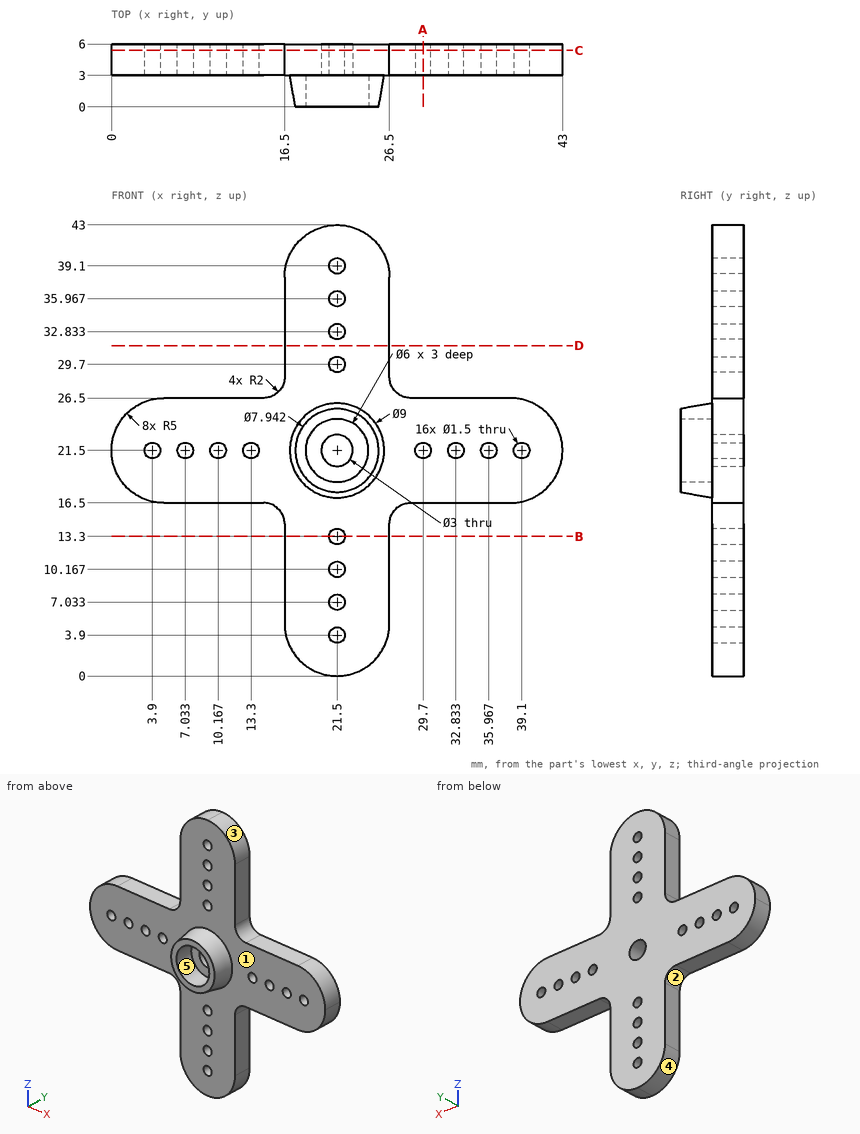
Verification items for this drawing (mm, ordinates from the low corner). A direction names the side the tool comes from. Round coordinates to 2 decimals unless told otherwise and drop trailing zeros. Write each loop counter-clockwise with the first axis right and the second up, starting at its lowest first coordinate (ties: lowest second). Pieces come first, ordered by that corner, then holes. Notation, with made-up numbers: M -8,0.5 L 29,0.5 A22 cw 29,31.5 Z; hole C 72.25,-11 d4. An arc over 180 degrees is marked long. Write item = value, one per line. Start each with the question number.
1. Gauge pin test, flat ends, axial feed: pin 1 (2 mm diameter, centred on y = 1.5, z = 35, fed in from -X); pin 2 (0.9 mm diameter, centred on y = 5, z = 10.5, fed in from +X); pin 3 (21.5 mm diameter, centred on x = 22, z = 18, fed in from -Y); pin 4 (5 mm diameter, centred on x = 21.5, z = 21.5, fed in from -Y). Record the tip position at first contact, or that the pin passes through.
2. Section check C-C, the plane y = 5.4. State how many separate pieces and enclosed holes the cut face has, then the cut area to 3 significant figures.
3. Section check A-A, the plane x = 29.7. Record the cut outline in (y, z), then the cut area to 3 significant figures.
4. Tool access check on the marked faces 1 and 2. Record the directions out of +Z, -Z, +X, -X, +Y, -Y that give a thin tool (end or side, any length) a straight path to the whole face; none if there is none.
5. Release check for a two-part mould opening along X. For the marked faces 3, 4 and 5 record: pulls with the +X half, pulls with the -X half, needs draft (parallel to the pull), parting line crosses it, or undercut.
6. Section check D-D, the plane z = 31.5. Record the cut outline in (x, y), then the cut area to 3 significant figures.
7. Section check B-B, the plane z = 13.3. Record the cut outline in (x, y), then the cut area to 3 significant figures.
8. Scan lines: line 1 (Y direction, x = 27, z = 19.5); line 2 (Z direction, x = 20.5, y = 5.3); line 3 (Z direction, x = 39.1, y = 5.2). Record each from-to range of solid material in increasing order. Write a range as [from, to].
Results found:
q1.pin_1 = through
q1.pin_2 = 26.5
q1.pin_3 = 0
q1.pin_4 = 3
q2.separate_pieces = 1
q2.enclosed_holes = 17
q2.area = 685 mm^2
q3.outline = M 3,16.5 L 6,16.5 L 6,20.75 L 3,20.75 Z; M 3,22.25 L 6,22.25 L 6,26.5 L 3,26.5 Z
q3.area = 25.5 mm^2
q4.face_1 = -Y
q4.face_2 = -Z, -X, +Y, -Y
q5.face_3 = pulls with the +X half
q5.face_4 = pulls with the -X half
q5.face_5 = undercut
q6.outline = M 16.5,3 L 26.5,3 L 26.5,6 L 16.5,6 Z
q6.area = 30.0 mm^2
q7.outline = M 16.5,3 L 20.75,3 L 20.75,6 L 16.5,6 Z; M 22.25,3 L 26.5,3 L 26.5,6 L 22.25,6 Z
q7.area = 25.5 mm^2
q8.line_1 = [3, 6]
q8.line_2 = [0.1, 20.38], [22.62, 42.9]
q8.line_3 = [16.62, 20.75], [22.25, 26.38]
